```python
from build123d import *

# Parameters (mm, degrees)
BOX003_W                 = 220
BOX003_H                 = 2.5
BOX003_DEPTH             = 3
EXTRUDE001_DEPTH         = 10
BOX002_W                 = 220
BOX002_H                 = 113
BOX002_DEPTH             = 8
BOX001_W                 = 32
BOX001_H                 = 6
BOX001_DEPTH             = 6
PRISM003_DEPTH           = 6
PRISM003_PLACEMENT_ANGLE = 30
PRISM002_DEPTH           = 6
PRISM002_PLACEMENT_ANGLE = 30


with BuildPart() as cube003:
    # Box003 → Box003 (new body)
    with BuildSketch(Plane(origin=(-110, 2, 0), x_dir=(1, 0, 0), z_dir=(0, 0, 1))):
        with Locations((110, 1.25)):
            Rectangle(BOX003_W, BOX003_H)
    extrude(amount=BOX003_DEPTH)


with BuildPart() as extrude001:
    # Sketch002 → Extrude001 (new body)
    with BuildSketch(Plane.XY):
        Polygon((-95, 0), (95, 0), (85, 61), (-85, 61), align=None)
    extrude(amount=EXTRUDE001_DEPTH)


with BuildPart() as obj1:
    # Box002 → Box002 (new body)
    with BuildSketch(Plane(origin=(-110, -15, 0), x_dir=(1, 0, 0), z_dir=(0, 0, 1))):
        with Locations((110, 56.5)):
            Rectangle(BOX002_W, BOX002_H)
    extrude(amount=BOX002_DEPTH)

    # Cut002: cut Extrude001
    add(extrude001.part, mode=Mode.SUBTRACT)


with BuildPart() as cube001:
    # Box001 → Box001 (new body)
    with BuildSketch(Plane(origin=(-16, 55, 0), x_dir=(1, 0, 0), z_dir=(0, 0, 1))):
        with Locations((16, 3)):
            Rectangle(BOX001_W, BOX001_H)
    extrude(amount=BOX001_DEPTH)


with BuildPart() as prism003:
    # Prism003 → Prism003 (new body)
    with BuildSketch(Plane.XY):
        Polygon((45, 0), (-22.5, 38.971143), (-22.5, -38.971143), align=None)
    extrude(amount=PRISM003_DEPTH)


with BuildPart() as prism003_1:
    # Prism003 placement: moved
    add(prism003.part.moved(Location((0, 23, 0))).rotate(Axis((0, 23, 0), (0, 0, -1)), PRISM003_PLACEMENT_ANGLE))


with BuildPart() as obj2:
    # Prism002 → Prism002 (new body)
    with BuildSketch(Plane.XY):
        Polygon((60, 0), (-30, 51.961524), (-30, -51.961524), align=None)
    extrude(amount=PRISM002_DEPTH)


with BuildPart() as obj2_1:
    # Prism002 placement: moved
    add(obj2.part.moved(Location((0, 23, 0))).rotate(Axis((0, 23, 0), (0, 0, -1)), PRISM002_PLACEMENT_ANGLE))

    # Cut001: cut Prism003
    add(prism003_1.part, mode=Mode.SUBTRACT)


with BuildPart() as obj2_2:
    # Cut001 placement: moved
    add(obj2_1.part.moved(Location((0, 7, 0))))

    # Fusion: union Cube001
    add(cube001.part)

    # Cut003: cut obj1
    add(obj1.part, mode=Mode.SUBTRACT)

    # Cut004: cut Cube003
    add(cube003.part, mode=Mode.SUBTRACT)


solid = obj2_2.part
```
Build history of the part. All positions in model axes, mm. A direction names the side the tool comes from. Round coordinates to 2 decimals unless told otherwise and drop trailing zeros. Write each loop counter-clockwise with the first axis right and the second up, starting at its lowest first coordinate (ties: lowest second). Pieces come first, ordered by that corner, then holes.
1) 3-axis set-ups, long thin cutter, end or side, ignore diameter. For faces 1 (the flat face through (-1, 2, 1)), 2 (the flat face through (0, 55, 3)), 3 (the flat face through (0, 61, 3)): which of +Z, -Z, +X, -X, +Y, -Y reach the whole face in a straight line?
2) Band-saw the part on C-C, the plane y = 43.5. List the corners of the cut face in (x, z).
3) Band-saw the part on A-A, the plane z = 4.7. List the corners of the cut face in (x, y).
4) Band-saw the part on D-D, the plane x = -28. List the corners of the cut face in (y, z).
5) Mould opens along Y. For faces 4 (the flat face through (-4, 1, 0)), 5 (the flat face through (-1, 7.5, 3)), 6 (the flat face through (34.6, 30.07, 2.96)) say: +Y half, -Y half, draft (parallel to the pull), parting line (faces both ways), or undercut.
6) Pin check, flat tips, straight feed: pin 1 (1.5 mm diameter, centred on y = 9, z = 3.5, fed in from -X); pin 2 (2.5 mm diameter, centred on x = 23.5, z = 2, fed in from +Y); pin 3 (3 mm diameter, centred on x = 37.5, z = 4.5, fed in from +Y); pin 4 (12 mm diameter, centred on x = 5, y = 47, fed in from -Z). Stop position of each tip, or through.
7) Band-saw the part on B-B, the plane x = 3. List the corners of the cut face in (y, z).
8) Drill centre lines: probe 1 along Y at (x, z) = (-9.5, 3.1); probe 2 along Y at (x, z) = (-4.5, 0.7); probe 3 along Y at (x, z) = (21, 2.2). Where is each one in solid material? Low to high.
Ans:
1. face 1: -Z, +X, -X
1. face 2: +Z, -Z
1. face 3: +Z, -Z, +X, -X, +Y
2. outline: (-26.85, 0) - (-18.19, 0) - (-18.19, 6) - (-26.85, 6) - close; (18.19, 0) - (26.85, 0) - (26.85, 6) - (18.19, 6) - close
3. outline: (-51.96, 0) - (51.96, 0) - (16.74, 61) - (-16.74, 61) - close; hole (-38.97, 7.5) - (38.97, 7.5) - (11.55, 55) - (-11.55, 55) - close
4. outline: (0, 0) - (2, 0) - (2, 3) - (4.5, 3) - (4.5, 0) - (7.5, 0) - (7.5, 6) - (0, 6) - close; (26.5, 0) - (41.5, 0) - (41.5, 6) - (26.5, 6) - close
5. face 4: draft
5. face 5: undercut
5. face 6: +Y half
6. pin 1: stops at x = -47.2
6. pin 2: stops at y = 51.46
6. pin 3: stops at y = 27.65
6. pin 4: passes through
7. outline: (0, 0) - (2, 0) - (2, 3) - (4.5, 3) - (4.5, 0) - (7.5, 0) - (7.5, 6) - (0, 6) - close; (55, 0) - (61, 0) - (61, 6) - (55, 6) - close
8. probe 1: y = 0 to 7.5, 55 to 61
8. probe 2: y = 0 to 2, 4.5 to 7.5, 55 to 61
8. probe 3: y = 0 to 2, 4.5 to 7.5, 38.63 to 53.63
